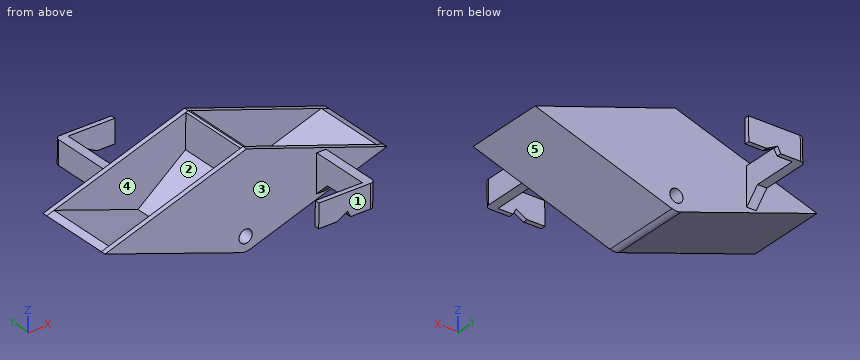
from build123d import *

# Parameters (mm, degrees)
PAD023_DEPTH        = 15
SKETCH047_R         = 1.4
POCKET020_DEPTH     = 15
PAD018_DEPTH        = 15
PAD020_DEPTH        = 1
PAD019_DEPTH        = 1
SKETCH049_R         = 1.4
POCKET023_DEPTH     = 17.001
PAD022_DEPTH        = 5
PAD021_DEPTH        = 5
CHAMFER009_SIZE     = 3
CHAMFER010_SIZE     = 3
FILLET014_R         = 1
FILLET013_R         = 1
POCKET022_DEPTH     = 1
POCKET021_DEPTH     = 1
BODY007_PITCH_ANGLE = 0.7


with BuildPart() as part:
    # Sketch051 → Pad023 (new body)
    with BuildSketch(Plane.XZ.offset(7.5)):
        with BuildLine():
            Line((0.962959, 0.158748), (30, 10))
            Line((30, 10), (28.432297, 10.524546))
            Line((28.432297, 10.524546), (10.5, 4.446921))
            Line((0, 13), (10.5, 4.446921))
            Line((0, 13), (-10.5, 4.446921))
            Line((-28.432297, 10.524546), (-10.5, 4.446921))
            Line((-30, 10), (-28.432297, 10.524546))
            Line((-0.962959, 0.158748), (-30, 10))
            ThreePointArc((-0.962959, 0.158748), (0, 0), (0.962959, 0.158748))
        make_face()
    extrude(amount=-PAD023_DEPTH)

    # Sketch047 → Pocket020 (cut)
    with BuildSketch(Plane.XZ.offset(7.5)):
        with Locations((0, 3)):
            Circle(SKETCH047_R)
    extrude(amount=-POCKET020_DEPTH, mode=Mode.SUBTRACT)

    # Sketch054 (on Face4 of Pocket020) → Pad018 (join)
    with BuildSketch(Plane.XZ.offset(7.5)):
        with BuildLine():
            Line((-0.5, 5.95804), (-0.5, 19.831731))
            Line((-0.5, 19.831731), (0, 20))
            Line((0, 20), (0.5, 19.831731))
            Line((0.5, 19.831731), (0.5, 5.95804))
            ThreePointArc((0.5, 5.95804), (0, 6), (-0.5, 5.95804))
        make_face()
    extrude(amount=-PAD018_DEPTH)

    # Sketch050 (on Face4 of Pad018) → Pad020 (join)
    with BuildSketch(Plane.XZ.offset(7.5)):
        with BuildLine():
            ThreePointArc((-0.962959, 0.158748), (0, 0), (0.962959, 0.158748))
            Line((30, 10), (0.962959, 0.158748))
            Line((0, 20), (30, 10))
            Line((-30, 10), (0, 20))
            Line((-0.962959, 0.158748), (-30, 10))
        make_face()
    extrude(amount=PAD020_DEPTH)

    # Sketch053 (on Face4 of Pad018) → Pad019 (join)
    with BuildSketch(Plane.XZ.offset(-7.5)):
        with BuildLine():
            ThreePointArc((-0.962959, 0.158748), (0, 0), (0.962959, 0.158748))
            Line((30, 10), (0.962959, 0.158748))
            Line((0, 20), (30, 10))
            Line((-30, 10), (0, 20))
            Line((-0.962959, 0.158748), (-30, 10))
        make_face()
    extrude(amount=-PAD019_DEPTH)

    # Sketch049 (on Face12 of Pad019) → Pocket023 (cut, through all)
    with BuildSketch(Plane.XZ.offset(8.5)):
        with Locations((0, 3)):
            Circle(SKETCH049_R)
    extrude(amount=-POCKET023_DEPTH, mode=Mode.SUBTRACT)

    # Sketch048 → Pad022 (join)
    with BuildSketch(Plane.XY.offset(9)):
        Polygon((5, -21), (5, -22), (17, -22), (17, -8.5), (15, -8.5), (15, -21), align=None)
    extrude(amount=PAD022_DEPTH)

    # Sketch055 → Pad021 (join)
    with BuildSketch(Plane(origin=(0, 0, 9), x_dir=(-1, 0, 0), z_dir=(0, 0, 1))):
        Polygon((5, -21), (5, -22), (17, -22), (17, -8.5), (15, -8.5), (15, -21), align=None)
    extrude(amount=PAD021_DEPTH)

    # Chamfer009
    chamfer009_edges = [part.edges().sort_by_distance(p)[0] for p in [
        (16, -8.5, 9),
    ]]
    chamfer(chamfer009_edges, length=CHAMFER009_SIZE)

    # Chamfer010
    chamfer010_edges = [part.edges().sort_by_distance(p)[0] for p in [
        (-16, 8.5, 9),
    ]]
    chamfer(chamfer010_edges, length=CHAMFER010_SIZE)

    # Fillet014
    fillet014_edges = [part.edges().sort_by_distance(p)[0] for p in [
        (17, -22, 11.5),
    ]]
    fillet(fillet014_edges, radius=FILLET014_R)

    # Fillet013
    fillet013_edges = [part.edges().sort_by_distance(p)[0] for p in [
        (-17, 22, 11.5),
    ]]
    fillet(fillet013_edges, radius=FILLET013_R)

    # Sketch056 (on Face52 of Fillet013) → Pocket022 (cut)
    with BuildSketch(Plane.XZ.offset(22)):
        Polygon((8.8, 9), (11.138789, 10.243556), (11.8, 9), align=None)
    extrude(amount=-POCKET022_DEPTH, mode=Mode.SUBTRACT)

    # Sketch052 (on Face7 of Pocket022) → Pocket021 (cut)
    with BuildSketch(Plane(origin=(0, 22, 0), x_dir=(1, 0, 0), z_dir=(0, 1, 0))):
        Polygon((-11.8, -9), (-11.138789, -10.243556), (-8.8, -9), align=None)
    extrude(amount=-POCKET021_DEPTH, mode=Mode.SUBTRACT)


with BuildPart() as part_1:
    # Body007 pitch: moved
    add(part.part.rotate(Axis((0, 0, 0), (0, 1, 0)), BODY007_PITCH_ANGLE))


with BuildPart() as part_2:
    # Body007 placement: moved
    add(part_1.part.moved(Location((-0.036651, 0, 0.000224))))


solid = part_2.part
Verification items for the finished model (mm, model axes). Face numbers are marked on the shaded views. A direction names the side the tool comes from. Give positions to 0.01 mm unless a question says otherwise; leave off trailing zeros. Loops run counter-clockwise (first coordinate to the right, second up) from the corner with the lowest first, then second, coordinate; pieces in that order, holes last.
1. Cross-section at A-A on x = 7. Record the cut outline in (y, z), and give its area (3 significant figures).
Derived:
outline: (-22, 8.91) - (-21, 8.91) - (-21, 13.92) - (-22, 13.92) - close; (-8.5, 2.12) - (8.5, 2.12) - (8.5, 17.64) - (7.5, 17.64) - (7.5, 7.26) - (-7.5, 7.26) - (-7.5, 17.64) - (-8.5, 17.64) - close
area: 113 mm2
2. Go/stop test with flat-tipped pins: P1, Ø5.5, axis at x = -10, z = 10.5, coming from the -Y side; P2, Ø0.6, axis at x = -29, z = 10.5, coming from the +Y side; P3, Ø3, axis at y = 5.5, z = 15, coming from the +X side (3 decimals). Record where each tip stops, or that it passes through.
Derived:
P1: stops at y = -8.5
P2: stops at y = 8.5
P3: stops at x = 0.665
3. Tool access check on the marked faces 1 and 2. Record the directions out of +Z, -Z, +X, -X, +Y, -Y that give a thin tool (end or side, any length) a straight path to the whole face; none if there is none.
Derived:
face 1: +Z, -Z, +X, -X, -Y
face 2: +Z
4. Material ranges on probe 1 along Y at (x, z) = (-7, 9); probe 2 along Y at (x, z) = (7.5, 4); probe 3 along X at (y, z) = (2, 18.75), recorded low to high.
Derived:
probe 1: y = -8.5 to -7.5, 7.5 to 8.5
probe 2: y = -8.5 to 8.5
probe 3: x = -0.31 to 0.69
5. Cross-section at D-D on y = 10. Record the cut outline in (x, z), and give its area (3 significant figures).
Derived:
outline: (-16.94, 7.71) - (-14.94, 7.68) - (-14.86, 14.18) - (-16.86, 14.21) - close
area: 13.0 mm2
6. Cross-section at B-B on y = -2. Record the cut outline in (x, z).
Derived:
outline: (-29.91, 10.37) - (-1, 0.17) arc R3 ccw to (0.93, 0.15) - (30.08, 9.63) - (28.52, 10.18) - (10.52, 4.32) - (0.62, 12.59) - (0.71, 19.82) - (0.21, 20) - (-0.29, 19.84) - (-0.38, 12.6) - (-10.48, 4.58) - (-28.34, 10.87) - close; hole circle Ø2.8 at (0, 3)
7. Release check for a two-part mould opening along X. For the marked faces 3, 4 and 5 record: +X half, -X half, draft (parallel to the pull), parting line (faces both ways), or undercut.
Derived:
face 3: draft
face 4: undercut
face 5: +X half
8. Cross-section at C-C on x = -26. Record the cut outline in (y, z), and give its area (3 significant figures).
Derived:
outline: (-8.5, 8.99) - (8.5, 8.99) - (8.5, 11.62) - (7.5, 11.62) - (7.5, 10.05) - (-7.5, 10.05) - (-7.5, 11.62) - (-8.5, 11.62) - close
area: 21.2 mm2
